Model file for the job. Use its own axes, mm. Round coordinates to 2 decimals unless told otherwise and drop trailing zeros. Loops run counter-clockwise (first coordinate to the right, second up) from the corner with the lowest first, then second, coordinate; pieces in that order, holes last. Notation, with made-up numbers: M 61.5,61 L 82.5,61 A18 cw 82.5,75 Z; hole C 84,13.25 d4. An arc over 180 degrees is marked long. Use a Markdown table: item, result. Add a question column.
Item 1: Saw through at B-B on x = 100. Write the cut outline in (y, z).
Item 2: Pin check, flat tip, straight feed: P1, Ø19.5, axis at x = -100, y = 100, coming from the +Z side. Stop position of the tip, or through.
Item 3: Wall check: L1, parallel to Y at x = 100, z = 1.85; L2, parallel to Y at x = 130, z = 1.9. Give the ranges that are in metal, low to high. Write a range as from..to.
Item 4: Saw through at A-A on y = 130. Write the cut outline in (x, z), then the cut area to 3 significant figures.
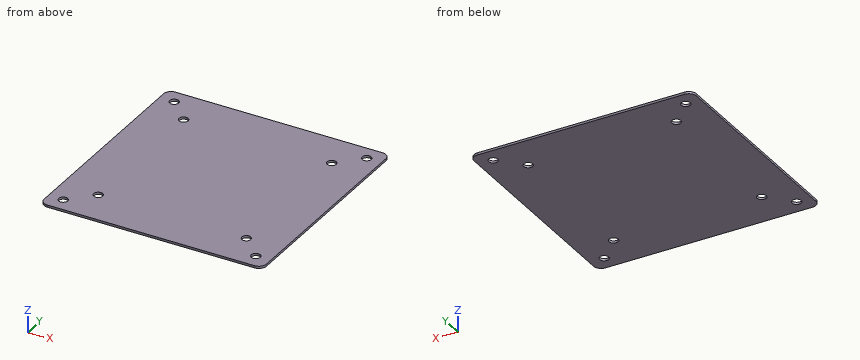
```python
from build123d import *

# Parameters (mm, degrees)
SKETCH1_W                        = 300
SKETCH1_H                        = 300
BOSS_EXTRUDE1_DEPTH              = 3
F_12_2_12_2_DIAMETER_HOLE1_D     = 12.2
F_12_2_12_2_DIAMETER_HOLE1_DEPTH = 23
F_12_2_12_2_DIAMETER_HOLE1_TIP   = 3.665249776
FILLET1_R                        = 10


with BuildPart() as part:
    # Sketch1 → Boss-Extrude1 (new body)
    with BuildSketch(Plane.XY):
        Rectangle(SKETCH1_W, SKETCH1_H)
    extrude(amount=BOSS_EXTRUDE1_DEPTH)

    # Ø12.2 (12.2) Diameter Hole1
    with Locations(Plane.XY.offset(3)):
        with Locations((-130, -130), (-100, -100), (130, -130), (100, -100), (130, 130), (-100, 100), (-130, 130), (100, 100)):
            Hole(F_12_2_12_2_DIAMETER_HOLE1_D / 2, depth=F_12_2_12_2_DIAMETER_HOLE1_DEPTH)
            with Locations((0, 0, -(F_12_2_12_2_DIAMETER_HOLE1_DEPTH + F_12_2_12_2_DIAMETER_HOLE1_TIP / 2))):  # 118° drill point
                Cone(0, F_12_2_12_2_DIAMETER_HOLE1_D / 2, F_12_2_12_2_DIAMETER_HOLE1_TIP, mode=Mode.SUBTRACT)

    # Fillet1
    fillet1_edges = [part.edges().sort_by_distance(p)[0] for p in [
        (150, -150, 1.5),
        (-150, -150, 1.5),
        (-150, 150, 1.5),
        (150, 150, 1.5),
    ]]
    fillet(fillet1_edges, radius=FILLET1_R)


solid = part.part
```
Entries:
| question | item | result |
|---|---|---|
| 1 | outline | M -150,0 L -106.1,0 L -106.1,3 L -150,3 Z; M -93.9,0 L 93.9,0 L 93.9,3 L -93.9,3 Z; M 106.1,0 L 150,0 L 150,3 L 106.1,3 Z |
| 2 | P1 | z = 3 |
| 3 | L1 | -150..-106.1, -93.9..93.9, 106.1..150 |
| 3 | L2 | -150..-136.1, -123.9..123.9, 136.1..150 |
| 4 | outline | M -150,0 L -136.1,0 L -136.1,3 L -150,3 Z; M -123.9,0 L 123.9,0 L 123.9,3 L -123.9,3 Z; M 136.1,0 L 150,0 L 150,3 L 136.1,3 Z |
| 4 | area | 827 mm2 |
